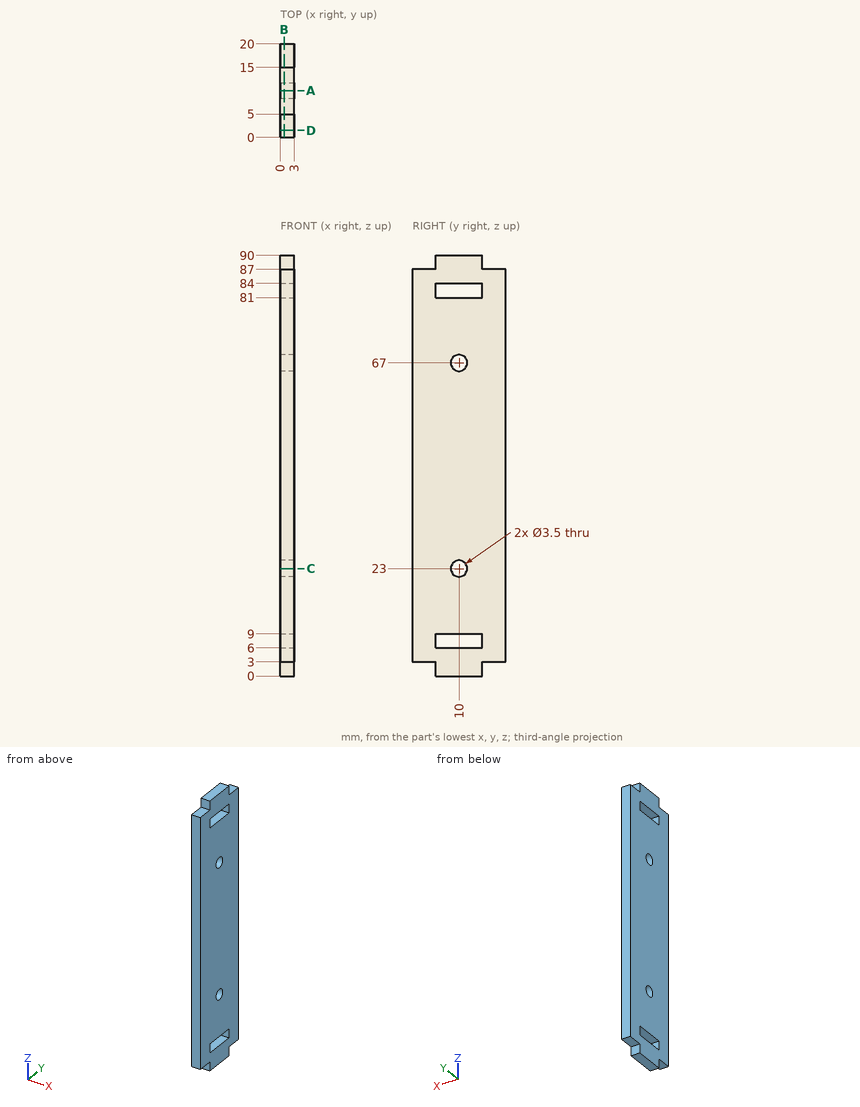
Answer from the drawing. Dimensions are ordinates in mm from the lowest x, y and z of the part. Coordinates: 2 decimals unless noted, no trailing zeros. Write each loop counter-clockwise with the first axis right and the second up, starting at its lowest first coordinate (ties: lowest second). Pieces come first, ordered by that corner, then holes. Notation, with made-up numbers: M 79.25,78.5 L 109.25,78.5 A27 cw 109.25,111.5 Z; hole C 39,-10 d3. An arc over 180 degrees is marked long. Put each result on its own line as item: value. Start each with the question number.
1. A cutting plane is placed at B-B on x = 0.8. Write down the section's boundary in (y, z).
2. A cutting plane is placed at A-A on y = 10. Write down the section's boundary in (x, z).
3. Consider line 1 (Z direction, x = 0.75, y = 8); line 2 (Z direction, x = 1.4, y = 10); line 3 (Y direction, x = 1.5, z = 67). Determine where each line is inside the solid, lowest interval first. Write a range as from..to.
4. A cutting plane is placed at C-C on z = 23. Write down the section's boundary in (x, y), then the cut area to 3 significant figures.
5. A cutting plane is placed at D-D on y = 1.5. Write down the section's boundary in (x, z), then the cut area to 3 significant figures.
6. Flat-ended cylindrical pins translate along their axes: P1, Ø1.5, axis at x = 2, z = 88, coming from the +Y side; P2, Ø0.9, axis at x = 1.5, y = 17, coming from the +Z side; P3, Ø0.9, axis at x = 2, y = 1.5, coming from the -Z side; P4, Ø1.5, axis at x = 1.5, z = 60.5, coming from the -Y side. Find the tip coordinate at first contact, or state that the pin passes through.
Resolved:
1. outline: M 0,3 L 5,3 L 5,0 L 15,0 L 15,3 L 20,3 L 20,87 L 15,87 L 15,90 L 5,90 L 5,87 L 0,87 Z; hole M 5,6 L 15,6 L 15,9 L 5,9 Z; hole M 5,81 L 15,81 L 15,84 L 5,84 Z; hole C 10,23 d3.5; hole C 10,67 d3.5
2. outline: M 0,0 L 3,0 L 3,6 L 0,6 Z; M 0,9 L 3,9 L 3,21.25 L 0,21.25 Z; M 0,24.75 L 3,24.75 L 3,65.25 L 0,65.25 Z; M 0,68.75 L 3,68.75 L 3,81 L 0,81 Z; M 0,84 L 3,84 L 3,90 L 0,90 Z
3. line 1: z = 0..6, 9..81, 84..90
3. line 2: z = 0..6, 9..21.25, 24.75..65.25, 68.75..81, 84..90
3. line 3: y = 0..8.25, 11.75..20
4. outline: M 0,0 L 3,0 L 3,8.25 L 0,8.25 Z; M 0,11.75 L 3,11.75 L 3,20 L 0,20 Z
4. area: 49.5 mm2
5. outline: M 0,3 L 3,3 L 3,87 L 0,87 Z
5. area: 252 mm2
6. P1: stops at y = 15
6. P2: stops at z = 87
6. P3: stops at z = 3
6. P4: stops at y = 0
